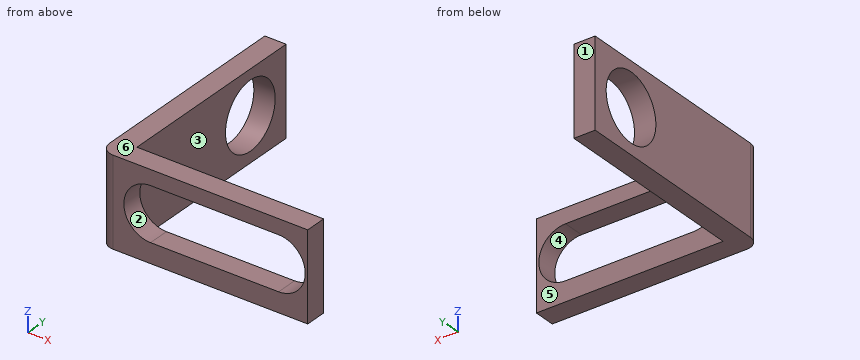
from build123d import *

# Parameters (mm, degrees)
BOSS_EXTRUDE1_DEPTH = 33
SKETCH2_R           = 12.5
CUT_EXTRUDE2_DEPTH  = 33
CUT_EXTRUDE10_DEPTH = 33


with BuildPart() as part:
    # Sketch1 → Boss-Extrude1 (new body)
    with BuildSketch(Plane.XY):
        with BuildLine():
            Line((0, 0), (0, 75))
            Line((0, 75), (8, 75))
            Line((8, 75), (8, 0))
            Line((8, 0), (78, 0))
            Line((78, 0), (78, -8))
            Line((78, -8), (5, -8))
            ThreePointArc((5, -8), (1.464466094, -6.535533906), (0, -3))
            Line((0, -3), (0, 0))
        make_face()
    extrude(amount=BOSS_EXTRUDE1_DEPTH)

    # Sketch2 → Cut-Extrude2 (cut)
    with BuildSketch(Plane(origin=(8, 0, 0), x_dir=(0, 0, -1), z_dir=(1, 0, 0))):
        with Locations(Location((-16.629694818, 57, 0), (0, 0, 90))):
            Circle(SKETCH2_R)
    extrude(amount=-CUT_EXTRUDE2_DEPTH, mode=Mode.SUBTRACT)

    # Sketch3 → Cut-Extrude10 (cut)
    with BuildSketch(Plane(origin=(0, 0, 0), x_dir=(1, 0, 0), z_dir=(0, 1, 0))):
        with BuildLine():
            Line((19.067260463, -7.366474126), (67.067260463, -7.366474126))
            ThreePointArc((67.067260463, -7.366474126), (77.067260463, -17.366474126), (67.067260463, -27.366474126))
            Line((67.067260463, -27.366474126), (19.067259653, -27.366474126))
            ThreePointArc((19.067259653, -27.366474126), (9.067259653, -17.366473721), (19.067260463, -7.366474126))
        make_face()
    extrude(amount=-CUT_EXTRUDE10_DEPTH, mode=Mode.SUBTRACT)


solid = part.part
Could you check a few things on this model? Use its own coordinates, in mm. Face numbers are marked on the shaded views. A direction names the side the tool comes from. Give positions to 0.01 mm unless a question says otherwise; leave off trailing zeros. Loops run counter-clockwise (first coordinate to the right, second up) from the corner with the lowest first, then second, coordinate; pieces in that order, holes last. Notation, with made-up numbers: (1, 69) -> (18, 69) arc R30 cw to (18, 102) -> close; hole circle Ø7 at (70, 8.25). An arc over 180 degrees is marked (long way). Return JSON: item names as keys, results as strings.
Item 1: We'd pull the mould along Z, two halves only. Please class the marked faces 4, 5 and 6: +Z half, -Z half, draft (parallel to the pull), parting line (faces both ways), or undercut.
Geometry results:
{"face 4": "undercut", "face 5": "draft", "face 6": "+Z half"}
Item 2: If we section it at B-B on y = 57: List the corners of the cut face in (x, z) for me, plus the area to 3 significant figures.
Geometry results:
{"outline": "(0, 0) -> (8, 0) -> (8, 4.13) -> (0, 4.13) -> close; (0, 29.13) -> (8, 29.13) -> (8, 33) -> (0, 33) -> close", "area": "64.0 mm²"}
Item 3: If we section it at A-A on x = 50: List the corners of the cut face in (y, z) for me.
Geometry results:
{"outline": "(-8, 0) -> (0, 0) -> (0, 7.37) -> (-8, 7.37) -> close; (-8, 27.37) -> (0, 27.37) -> (0, 33) -> (-8, 33) -> close"}
Item 4: I need wall thicknesses on L1, parallel to Z at x = 4, y = 57; L2, parallel to X at y = 25.5, z = 25.5; L3, parallel to Y at x = 23.5, z = 2.5. Which ranges of each line are inside material? Lowest first, please. Write a range as from..to.
Geometry results:
{"L1": "z = 0..4.13, 29.13..33", "L2": "x = 0..8", "L3": "y = -8..0"}
Item 5: If we section it at D-D on y = 5: List the corners of the cut face in (x, z) for me, plus the area to 3 significant figures.
Geometry results:
{"outline": "(0, 0) -> (8, 0) -> (8, 33) -> (0, 33) -> close", "area": "264 mm²"}
Item 6: If we section it at C-C on z = 18: List the corners of the cut face in (x, y) for me, plus the area to 3 significant figures.
Geometry results:
{"outline": "(0, -3) arc R5 ccw to (5, -8) -> (9.09, -8) -> (9.09, 0) -> (8, 0) -> (8, 44.58) -> (0, 44.58) -> close; (0, 69.42) -> (8, 69.42) -> (8, 75) -> (0, 75) -> close; (77.05, -8) -> (78, -8) -> (78, 0) -> (77.05, 0) -> close", "area": "476 mm²"}
Item 7: Which directions (+Z, -Z, +X, -X, +Y, -Y) give clear straight access to the entire face, cutting with the end or side of a thin tool? Please do the marked faces 1, 2 and 3.
Geometry results:
{"face 1": "+Z, -Z, +X, -X, +Y", "face 2": "+Y, -Y", "face 3": "+Z, -Z, +X, +Y"}
Item 8: I'm going to push flat-ended pins straight in: pin 1 (1.5 mm diameter, centred on y = 1, z = 21.5, fed in from +X); pin 2 (12 mm diameter, centred on x = 46, z = 7, fed in from +Y); pin 3 (6.5 mm diameter, centred on x = 46, y = -5.5, fed in from -Z). Where does each tip first touch, or does it pass through?
Geometry results:
{"pin 1": "stops at x = 8", "pin 2": "stops at y = 0", "pin 3": "stops at z = 0"}
